```python
from build123d import *

# Parameters (mm, degrees)
SKETCH1_R           = 40
BOSS_EXTRUDE1_DEPTH = 3
SKETCH2_R           = 27.5
CUT_EXTRUDE1_DEPTH  = 57.648036153
MOVE_FACE1_BY       = 0.3
SKETCH6_R           = 0.95
CUT_EXTRUDE8_DEPTH  = 57.632940944
CIRPATTERN3_COUNT   = 5
BOSS_EXTRUDE2_DEPTH = 8
CIRPATTERN4_COUNT   = 30


with BuildPart() as part:
    # Sketch1 → Boss-Extrude1 (new body)
    with BuildSketch(Plane.XY):
        Circle(SKETCH1_R)
    extrude(amount=BOSS_EXTRUDE1_DEPTH)

    # Sketch2 → Cut-Extrude1 (cut, through all)
    with BuildSketch(Plane.XY.offset(3)):
        Circle(SKETCH2_R)
    extrude(amount=-CUT_EXTRUDE1_DEPTH, mode=Mode.SUBTRACT)

    # Move Face1: a face moved inward by 0.3
    extrude(part.faces().sort_by_distance((0, -32, 0))[0], amount=MOVE_FACE1_BY, dir=(0, 0, 1), mode=Mode.SUBTRACT)

    # Sketch6 → Cut-Extrude8 (cut, through all)
    with BuildSketch(Plane(origin=(0, 0, 0.3), x_dir=(-1, 0, 0), z_dir=(0, 0, -1))):
        with Locations((11.467774385, 29.874573648)):
            Circle(SKETCH6_R)
    cut_extrude8 = extrude(amount=-CUT_EXTRUDE8_DEPTH, mode=Mode.SUBTRACT)

    # CirPattern3: Cut-Extrude8 ×5 about axis
    cirpattern3_axis = Axis((0, 0, 0), (0, 0, 1))
    for i in range(1, CIRPATTERN3_COUNT):
        add(cut_extrude8.rotate(cirpattern3_axis, i * 360 / CIRPATTERN3_COUNT), mode=Mode.SUBTRACT)

    # Sketch7 → Boss-Extrude2 (add)
    with BuildSketch(Plane.XY.offset(3)):
        with BuildLine():
            Line((-1.988766337, 37.947922321), (-2.09343825, 39.94518139))
            ThreePointArc((-2.09343825, 39.94518139), (0, 40), (2.09343825, 39.94518139))
            Line((2.09343825, 39.94518139), (1.988766337, 37.947922321))
            ThreePointArc((1.988766337, 37.947922321), (0, 38), (-1.988766337, 37.947922321))
        make_face()
    boss_extrude2 = extrude(amount=BOSS_EXTRUDE2_DEPTH)

    # CirPattern4: Boss-Extrude2 ×30 about axis
    cirpattern4_axis = Axis((0, 0, 0), (0, 0, 1))
    for i in range(1, CIRPATTERN4_COUNT):
        add(boss_extrude2.rotate(cirpattern4_axis, i * 360 / CIRPATTERN4_COUNT))


solid = part.part
```
CAD build for the part. Positions are in the model's coordinates, mm. A direction names the side the tool comes from. Round coordinates to 2 decimals unless told otherwise and drop trailing zeros. Order: outer loops, then holes, each group sorted by start corner. A loop starts at its lowest first (then second) coordinate and runs counter-clockwise, first axis right, second up.
Q1. Wall check: L1, parallel to Y at x = 0, z = 1.45; L2, parallel to Z at x = -29, y = -24; L3, parallel to Y at x = 21, z = 1.25. Give the ranges that are in metal, low to high.
Q2. Slice it at B-B (z = 7.75). State how many separate pieces and enclosed holes the cut face has, and give its area (3 significant figures).
Q3. Which spindle directions (+Z, -Z, +X, -X, +Y, -Y) get a long thin tool onto all of the face, cutting with end or side? Do faces 1 (the flat face through (-39, -4, 11)), 2 (the cylindrical face through (25.696, 19.671, 1.631)), 3 (the flat face through (-37.7, 10.1, 6.9)), 4 (the cylindrical face through (0, -38, 7)), 5 (the flat face through (17.7, -34.74, 6.94)). Say none if no direction does.
Q4. Drop flat-ended pins along their axis: pin 1 (2 mm diameter, centred on y = -6, z = 9, fed in from -X); pin 2 (3 mm diameter, centred on x = 24.87, y = 20.14, fed in from -Z); pin 3 (1 mm diameter, centred on y = 2.5, z = 5.5, fed in from -X); pin 4 (5 mm diameter, centred on x = 13.5, z = 1.5, fed in from +Y). Give the stop position or say it passes through.
Q5. Two-plate mould, pull along Y, no slides. Class faces 6 (the flat face through (13.971, 36.397, 6.944)), 7 (the flat face through (37, 12, 11)), 8 (the cylindrical face through (-11.262, 28.947, 1.631)): pulls with the +Y half, pulls with the -Y half, needs draft (parallel to the pull), parting line crosses it, or undercut.
Q6. Slice it at A-A (x = 0). Write the cut outline in (y, z).
Results below:
1. L1: y = -40 to -27.5, 27.5 to 40
1. L2: z = 0.3 to 3
1. L3: y = -34.04 to -17.76, 17.76 to 34.04
2. separate pieces: 30
2. enclosed holes: 0
2. area: 245 mm2
3. face 1: +Z, +X, -X, +Y, -Y
3. face 2: +Z, -Z
3. face 3: +Z, -X
3. face 4: +Z
3. face 5: +Z, +X
4. pin 1: stops at x = -39.69
4. pin 2: stops at z = 0.3
4. pin 3: stops at x = -39.95
4. pin 4: stops at y = 38.46
5. face 6: pulls with the +Y half
5. face 7: needs draft
5. face 8: undercut
6. outline: (-40, 0.3) - (-27.5, 0.3) - (-27.5, 3) - (-38, 3) - (-38, 11) - (-40, 11) - close; (27.5, 0.3) - (40, 0.3) - (40, 11) - (38, 11) - (38, 3) - (27.5, 3) - close
